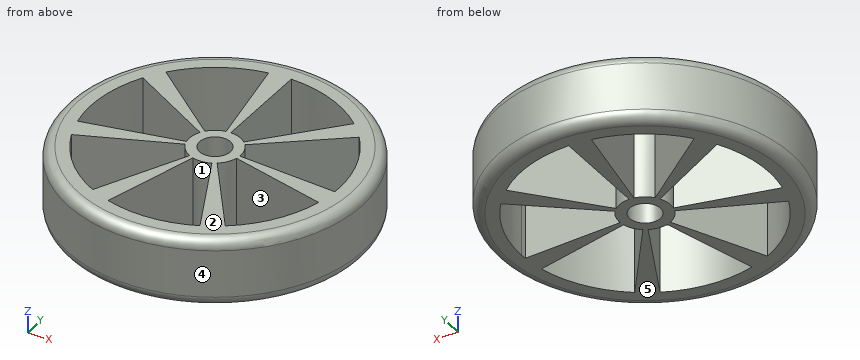
```python
from build123d import *

# Parameters (mm, degrees)
SKETCH1_R           = 14.3
BOSS_EXTRUDE1_DEPTH = 6.6
FILLET1_R           = 1
FILLET2_R           = 1
CUT_EXTRUDE1_DEPTH  = 10
SKETCH3_R           = 1.5
CUT_EXTRUDE2_DEPTH  = 10


with BuildPart() as part:
    # Sketch1 → Boss-Extrude1 (new body)
    with BuildSketch(Plane.XY):
        Circle(SKETCH1_R)
    extrude(amount=BOSS_EXTRUDE1_DEPTH)

    # Fillet1
    fillet1_edges = [part.edges().sort_by_distance(p)[0] for p in [
        (-14.3, 0, 6.6),
    ]]
    fillet(fillet1_edges, radius=FILLET1_R)

    # Fillet2
    fillet2_edges = [part.edges().sort_by_distance(p)[0] for p in [
        (-14.3, 0, 0),
    ]]
    fillet(fillet2_edges, radius=FILLET2_R)

    # Sketch2 → Cut-Extrude1 (cut)
    with BuildSketch(Plane.XY.offset(6.6)):
        with BuildLine():
            ThreePointArc((-1.954578706, 1.558724505), (-1.276893228, 2.149312375), (-0.434120444, 2.462019383))
            Line((-0.434120444, 2.462019383), (-2.095426853, 11.883756218))
            ThreePointArc((-2.095426853, 11.883756218), (-6.163350277, 10.374371736), (-9.434424854, 7.52370276))
            Line((-9.434424854, 7.52370276), (-1.954578706, 1.558724505))
        make_face()
        with BuildLine():
            ThreePointArc((-2.43731978, -0.556302335), (-2.476529986, 0.341759021), (-2.195553933, 1.195634947))
            Line((-2.195553933, 1.195634947), (-10.597572015, 5.771130126))
            ThreePointArc((-10.597572015, 5.771130126), (-11.953796477, 1.649613694), (-11.764535365, -2.685178426))
            Line((-11.764535365, -2.685178426), (-2.43731978, -0.556302335))
        make_face()
        with BuildLine():
            ThreePointArc((-1.084709348, -2.25242217), (-1.811289152, -1.723145846), (-2.30369053, -0.971086991))
            Line((-2.30369053, -0.971086991), (-11.119529298, -4.68727466))
            ThreePointArc((-11.119529298, -4.68727466), (-8.742790117, -8.317337105), (-5.235710794, -10.87206549))
            Line((-5.235710794, -10.87206549), (-1.084709348, -2.25242217))
        make_face()
        with BuildLine():
            Line((5.235710794, -10.87206549), (1.084709348, -2.25242217))
            ThreePointArc((1.084709348, -2.25242217), (0.217889357, -2.490486745), (-0.67710117, -2.406560617))
            Line((-0.67710117, -2.406560617), (-3.268254223, -11.616066024))
            ThreePointArc((-3.268254223, -11.616066024), (1.051715522, -12.021163422), (5.235710794, -10.87206549))
        make_face()
        with BuildLine():
            Line((11.764535365, -2.685178426), (2.43731978, -0.556302335))
            ThreePointArc((2.43731978, -0.556302335), (2.082992736, -1.382440328), (1.459359181, -2.029845014))
            Line((1.459359181, -2.029845014), (7.044082942, -9.797722748))
            ThreePointArc((7.044082942, -9.797722748), (10.054257921, -6.672808494), (11.764535365, -2.685178426))
        make_face()
        with BuildLine():
            Line((9.434424854, 7.52370276), (1.954578706, 1.558724505))
            ThreePointArc((1.954578706, 1.558724505), (2.359708326, 0.825697655), (2.5, 0))
            ThreePointArc((2.5, 0), (2.499222955, -0.062326729), (2.496892303, -0.124614714))
            Line((2.496892303, -0.124614714), (12.052081979, -0.601494405))
            ThreePointArc((12.052081979, -0.601494405), (12.063331646, -0.300840709), (12.067082313, 0))
            ThreePointArc((12.067082313, 0), (11.389917841, 3.985504627), (9.434424854, 7.52370276))
        make_face()
        with BuildLine():
            Line((0, 12.067082313), (0, 2.5))
            ThreePointArc((0, 2.5), (0.884270174, 2.338389672), (1.654214594, 1.874453007))
            Line((1.654214594, 1.874453007), (7.984617468, 9.047671493))
            ThreePointArc((7.984617468, 9.047671493), (4.268224391, 11.287016262), (0, 12.067082313))
        make_face()
    extrude(amount=-CUT_EXTRUDE1_DEPTH, mode=Mode.SUBTRACT)

    # Sketch3 → Cut-Extrude2 (cut)
    with BuildSketch(Plane.XY.offset(6.6)):
        Circle(SKETCH3_R)
    extrude(amount=-CUT_EXTRUDE2_DEPTH, mode=Mode.SUBTRACT)


solid = part.part
```
Input: part model. Units: mm. Frame: model coordinates. Face numbers are marked on the shaded views. A direction names the side the tool comes from. Give positions to 0.01 mm unless a question says otherwise; leave off trailing zeros. Use a Markdown table: item, result.
Q1. Access query for the marked faces 1 and 2. Directions: +Z, -Z, +X, -X, +Y, -Y. A direction counts if a zero-diameter tool reaches every point of the face in a straight line with its end or side. Return the directions, or none.
Entries:
| item | result |
|---|---|
| face 1 | +Z, -Z |
| face 2 | +Z, +X, -X, +Y, -Y |
Q2. Ray query, probe 1 along X at (y, z) = (-6.5, 3); probe 2 along Y at (x, z) = (-9.75, 2.75); probe 3 along Y at (x, z) = (-8.25, 2.5). Return the intervals inside material, ascending. Write a range as from..to.
Entries:
| item | result |
|---|---|
| probe 1 | x = -12.74..-10.17, -3.13..-1.83, 3.13..4.67, 10.17..12.74 |
| probe 2 | y = -10.46..-7.11, -4.11..-2.23, 5.31..10.46 |
| probe 3 | y = -11.68..-8.81, -3.48..-1.88, 4.49..6.58, 8.81..11.68 |
Q3. Pull-direction query (X, two-part tool) for the marked faces 3, 4 and 5; classes: pulls with the +X half, pulls with the -X half, needs draft (parallel to the pull), parting line crosses it, or undercut.
Entries:
| item | result |
|---|---|
| face 3 | undercut |
| face 4 | parting line crosses it |
| face 5 | needs draft |
Q4. First-contact query: P1, Ø1.5, axis at y = 4, z = 1, coming from the -X side; P2, Ø2.5, axis at x = 0, y = 0, coming from the +Z side; P3, Ø3, axis at x = -6, z = 2.5, coming from the -Y side; P4, Ø2, axis at y = 7.5, z = 2, coming from the +X side. Flat tips, straight axial feed; report the tip coordinate or a pass-through.
Entries:
| item | result |
|---|---|
| P1 | stops at x = -13.93 |
| P2 | passes through |
| P3 | stops at y = -13.57 |
| P4 | stops at x = 12.74 |
Q5. Section query A-A, the plane z = 2.25. State how many separate pieces and enclosed holes the cut face has, plus the area to 3 significant figures.
Entries:
| item | result |
|---|---|
| separate pieces | 1 |
| enclosed holes | 8 |
| area | 283 mm² |
